from build123d import *

# Parameters (mm, degrees)
SKETCH1_R                = 6.5
SKETCH1_R_2              = 4.5
BOSS_EXTRUDE1_DEPTH      = 15
BOSS_EXTRUDE2_DEPTH      = 2
BOSS_EXTRUDE2_DEPTH_BACK = 3
SKETCH2_R                = 6.5
SKETCH2_R_2              = 3.223163269


with BuildPart() as part:
    # Sketch1 → Boss-Extrude1 (new body)
    with BuildSketch(Plane.XY):
        Circle(SKETCH1_R)
        Circle(SKETCH1_R_2, mode=Mode.SUBTRACT)
    extrude(amount=BOSS_EXTRUDE1_DEPTH)

    # Sketch2 → Boss-Extrude2 (add, two sides: drawn at the far end of the back side and taken through both)
    with BuildSketch(Plane(origin=(0, 0, 0), x_dir=(-1, 0, 0), z_dir=(0, 0, -1)).offset(-BOSS_EXTRUDE2_DEPTH_BACK)):
        Circle(SKETCH2_R)
        Circle(SKETCH2_R_2, mode=Mode.SUBTRACT)
    extrude(amount=BOSS_EXTRUDE2_DEPTH + BOSS_EXTRUDE2_DEPTH_BACK)


solid = part.part
Geometry: final body of the model. Coordinates: model frame, mm. A direction names the side the tool comes from. Give positions to 0.01 mm unless a question says otherwise; leave off trailing zeros. Order: outer loops, then holes, each group sorted by start corner. A loop starts at its lowest first (then second) coordinate and runs counter-clockwise, first axis right, second up. Notation, with made-up numbers: (71.25, -14) -> (111.25, -14) arc R21 ccw to (111.25, 20) -> close; hole circle Ø2 at (58.25, -1). An arc over 180 degrees is marked (long way). Put each result on its own line as item: value.
Q1. Material intervals for L1, parallel to Y at x = 0, z = 12.25; L2, parallel to Y at x = 0, z = 1.4, sorted ascending.
Here are the results:
L1: y = -6.5 to -4.5, 4.5 to 6.5
L2: y = -6.5 to -3.22, 3.22 to 6.5
Q2. Draft query along Y for faces 1 (the face through (2, 3, -2)), 2 (the face through (-0.59, 4.46, 8.92)). Return one class per face: released by +Y, released by -Y, zero draft, split by the parting line, or undercut.
Here are the results:
face 1: zero draft
face 2: undercut
Q3. Pin query (flat end, axial travel): pin 1 (1.5 mm diameter, centred on x = 1, z = 6, fed in from -Y); pin 2 (1.5 mm diameter, centred on x = 1, y = -2, fed in from -Z); pin 3 (5 mm diameter, centred on y = -3.5, z = 3, fed in from -X); pin 4 (1 mm diameter, centred on x = -3, z = 8, fed in from -Y). Return the tip coordinate at first contact, or that it passes through.
Here are the results:
pin 1: stops at y = -6.5
pin 2: passes through
pin 3: stops at x = -6.42
pin 4: stops at y = -6
Q4. Section D-D, the plane x = 3.5. Return loops of the section in (y, z), then the cut area to 3 significant figures.
Here are the results:
outline: (-5.48, -2) -> (5.48, -2) -> (5.48, 15) -> (2.83, 15) -> (2.83, 3) -> (-2.83, 3) -> (-2.83, 15) -> (-5.48, 15) -> close
area: 118 mm^2
Q5. Section A-A, the plane x = 0. Return loops of the section in (y, z), then the cut area to 3 significant figures.
Here are the results:
outline: (-6.5, -2) -> (-3.22, -2) -> (-3.22, 3) -> (-4.5, 3) -> (-4.5, 15) -> (-6.5, 15) -> close; (3.22, -2) -> (6.5, -2) -> (6.5, 15) -> (4.5, 15) -> (4.5, 3) -> (3.22, 3) -> close
area: 80.8 mm^2
Q6. Section B-B, the plane y = -0.5. Return loops of the section in (x, z), then the cut area to 3 significant figures.
Here are the results:
outline: (-6.48, -2) -> (-3.18, -2) -> (-3.18, 3) -> (-4.47, 3) -> (-4.47, 15) -> (-6.48, 15) -> close; (3.18, -2) -> (6.48, -2) -> (6.48, 15) -> (4.47, 15) -> (4.47, 3) -> (3.18, 3) -> close
area: 81.2 mm^2
Q7. Reachability of faces 3 (the face through (2.56, -1.96, 0.54)), 4 (the face through (-2, -3, 3)) from +Z, -Z, +X, -X, +Y, -Y: full face, straight path, thin tool, end or side. Return the list, or none.
Here are the results:
face 3: +Z, -Z
face 4: +Z
Q8. Section C-C, the plane z = 0.75. Return loops of the section in (x, y).
Here are the results:
outline: circle Ø13 at (0, 0); hole circle Ø6.45 at (0, 0)
